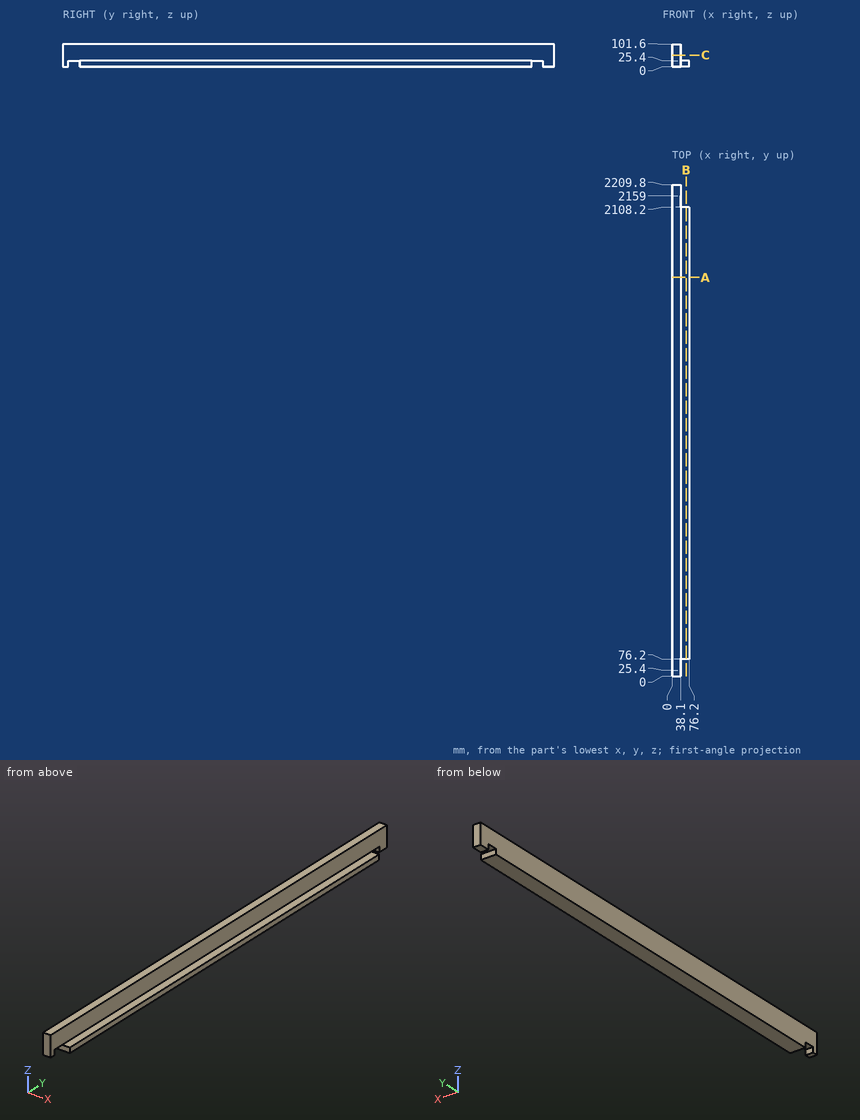
Check sheet for the drawn part. Datum: minimum x, y, z corner. Units: mm. Coordinates: 2 decimals unless noted, no trailing zeros. Order: outer loops, then holes, each group sorted by start corner. A loop starts at its lowest first (then second) coordinate and runs counter-clockwise, first axis right, second up. Notation, with made-up numbers: (44, 5.25) -> (53, 5.25) arc R8 cw to (53, 11.25) -> close; hole circle Ø11 at (1, 70.5). An arc over 180 degrees is marked (long way). Write each question's results on one line, items separated by ' | '. Start each with the question number.
1) Depth check by flat-ended pin: pin 1 (10 mm diameter, centred on y = 1772, z = 59.5, fed in from +X); pin 2 (11.5 mm diameter, centred on x = 58, y = 986.5, fed in from +Z); pin 3 (2 mm diameter, centred on x = 67, z = 18.5, fed in from +Y). Enter the tip coordinate at first touch or a pass-through.
2) Section check A-A (y = 1793). Enter the section's corners in (x, z), and give its area (3 significant figures).
3) Section check C-C (z = 52). Enter the section's corners in (x, y).
4) Section check B-B (x = 62.5). Enter the section's corners in (y, z), and give its area (3 significant figures).
5) Material ranges on line 1 along Y through (x, z) = (18, 25); line 2 along X through (y, z) = (1965, 54.5); line 3 along Y through (x, z) = (61, 24), recorded low to high.
Checked values:
1) pin 1: x = 38.1 | pin 2: z = 25.4 | pin 3: y = 2108.2
2) outline: (0, 0) -> (76.2, 0) -> (76.2, 25.4) -> (38.1, 25.4) -> (38.1, 101.6) -> (0, 101.6) -> close | area: 4,840 mm²
3) outline: (0, 0) -> (38.1, 0) -> (38.1, 2209.8) -> (0, 2209.8) -> close
4) outline: (76.2, 0) -> (2108.2, 0) -> (2108.2, 25.4) -> (76.2, 25.4) -> close | area: 51,600 mm²
5) line 1: 0 to 25.4, 76.2 to 2108.2, 2159 to 2209.8 | line 2: 0 to 38.1 | line 3: 76.2 to 2108.2
